from build123d import *

# Parameters (mm, degrees)
SKETCH_1_W          = 7
SKETCH_1_H          = 5
EXTRUDE_1_DEPTH     = 13
SKETCH_2_W          = 7
SKETCH_2_H          = 5
EXTRUDE_2_DEPTH     = 18.5
SKETCH_4_W          = 20
SKETCH_4_H          = 10
EXTRUDE_3_DEPTH     = 3
SKETCH_5_R          = 1.5
CUT_EXTRUDE_1_DEPTH = 34.559648389
FILLET_1_R          = 10
SKETCH_6_W          = 7
SKETCH_6_H          = 8
CUT_EXTRUDE_2_DEPTH = 0.1
CHAMFER_3_SIZE      = 2
CHAMFER_3_SIZE2     = 3


with BuildPart() as part:
    # 草图1 → 凸台-拉伸1 (new body)
    with BuildSketch(Plane(origin=(0, 0, 0), x_dir=(1, 0, 0), z_dir=(0, 1, 0))):
        Rectangle(SKETCH_1_W, SKETCH_1_H)
    extrude(amount=EXTRUDE_1_DEPTH)

    # 草图2 → 凸台-拉伸2 (add)
    with BuildSketch(Plane(origin=(0, 0, -2.5), x_dir=(-1, 0, 0), z_dir=(0, 0, -1))):
        with Locations((0, 10.5)):
            Rectangle(SKETCH_2_W, SKETCH_2_H)
    extrude(amount=EXTRUDE_2_DEPTH)

    # 草图4 → 凸台-拉伸3 (add)
    with BuildSketch(Plane(origin=(0, 0, -21), x_dir=(-1, 0, 0), z_dir=(0, 0, -1))):
        with Locations((0, 13)):
            Rectangle(SKETCH_4_W, SKETCH_4_H)
    extrude(amount=EXTRUDE_3_DEPTH)

    # 草图5 → 切除-拉伸1 (cut, through all)
    with BuildSketch(Plane(origin=(0, 0, -24), x_dir=(-1, 0, 0), z_dir=(0, 0, -1))):
        with Locations((-7, 13)):
            Circle(SKETCH_5_R)
        with Locations((7, 13)):
            Circle(SKETCH_5_R)
    extrude(amount=-CUT_EXTRUDE_1_DEPTH, mode=Mode.SUBTRACT)

    # 圆角1
    # the kernel refuses this fillet: 10 mm, written as the material it adds along each edge
    with BuildSketch(Plane(origin=(3.5, 13, -21), x_dir=(0, 1, 0), z_dir=(-1, 0, 0))) as fillet_1_piece_1:
        with BuildLine():
            CenterArc((10, -8.660254038), FILLET_1_R, 120, 60)
            Line((0, -8.660254038), (-0.2, -8.660254038))
            Line((-0.2, -8.660254038), (-0.2, 0))
            Line((-0.2, 0), (0, 0.2))
            ThreePointArc((0, 0.2), (2.5, 0.2), (4.9, 0.173205081))
            Line((4.9, 0.173205081), (5, 0))
        make_face()
    extrude(amount=7)

    # 草图6 → 切除-拉伸2 (cut)
    with BuildSketch(Plane(origin=(0, 0, -2.5), x_dir=(-1, 0, 0), z_dir=(0, 0, -1))):
        with Locations((0, 4)):
            Rectangle(SKETCH_6_W, SKETCH_6_H)
    extrude(amount=-CUT_EXTRUDE_2_DEPTH, mode=Mode.SUBTRACT)

    # 倒角3
    chamfer_3_edges = [part.edges().sort_by_distance(p)[0] for p in [
        (3.5, 0, 0.05),
        (-3.5, 0, 0.05),
    ]]
    chamfer_3_side = [part.faces().sort_by_distance(p)[0] for p in [
        (0, 0, 0.05),
    ]]
    chamfer(chamfer_3_edges, length=CHAMFER_3_SIZE, length2=CHAMFER_3_SIZE2, reference=chamfer_3_side[0])


solid = part.part
CAD build for the part. Positions are in the model's coordinates, mm. A direction names the side the tool comes from. Round coordinates to 2 decimals unless told otherwise and drop trailing zeros. Loops run counter-clockwise (first coordinate to the right, second up) from the corner with the lowest first, then second, coordinate; pieces in that order, holes last. Notation, with made-up numbers: (-34.5, 47.5) - (-2.5, 47.5) arc R21 ccw to (-2.5, 85.5) - close; hole circle Ø5 at (48, 38.25). An arc over 180 degrees is marked (long way). Put each result on its own line as item: value.
1. Two-plate mould, pull along X, no slides. Class faces 1 (the flat face through (2.5, 1.5, 0.1)), 2 (the flat face through (0, 4, -2.4)), 3 (the cylindrical face through (8.5, 13.07, -22.52)): released by +X, released by -X, zero draft, split by the parting line, or undercut.
Geometry check:
face 1: released by +X
face 2: zero draft
face 3: undercut
2. Slice it at C-C on y = 10. List the corners of the cut face in (x, z), and give its area (4 significant figures).
Geometry check:
outline: (-10, -24) - (10, -24) - (10, -21) - (3.5, -21) - (3.5, 2.5) - (-3.5, 2.5) - (-3.5, -21) - (-10, -21) - close
area: 224.5 mm²
3. Slice it at D-D on x = -2. List the corners of the cut face in (y, z), and give its area (3 significant figures).
Geometry check:
outline: (0.75, -2.4) - (8, -2.4) - (8, -24) - (18, -24) - (18, -21) arc R10 cw to (13, -12.34) - (13, 2.5) - (0.75, 2.5) - close
area: 196 mm²
4. 3-axis set-ups, long thin cutter, end or side, ignore diameter. For faces 4 (the flat face through (-3.5, 11, -9)), 5 (the flat face through (3.5, 11, -9)), 6 (the flat face through (0, 8, -15)), 7 (the flat face through (0, 13, -5)), 8 (the cylindrical face through (-5.5, 13.07, -22.52)): which of +Z, -Z, +X, -X, +Y, -Y reach the whole face in a straight line?
Geometry check:
face 4: +Z, -X, +Y, -Y
face 5: +Z, +X, +Y, -Y
face 6: -Z, +X, -X, -Y
face 7: +Z, +X, -X, +Y
face 8: +Z, -Z
5. Slice it at B-B on z = -22.25. List the corners of the cut face in (x, y).
Geometry check:
outline: (-10, 8) - (10, 8) - (10, 18) - (-10, 18) - close; hole circle Ø3 at (-7, 13); hole circle Ø3 at (7, 13)
6. Pin check, flat tips, straight feed: P1, Ø6, axis at y = 5, z = -4.5, coming from the -X side; P2, Ø6, axis at x = -3, z = -11, coming from the -Y side; P3, Ø3.5, axis at x = 1, y = 4.5, coming from the -Z side. Stop position of each tip, or through.
Geometry check:
P1: x = -3.5
P2: y = 8
P3: z = -2.4
7. Wall check: line 1 (Y direction, x = 7, z = -22.1); line 2 (X direction, y = 12.25, z = -3.25); line 3 (Z direction, x = 6, y = 10.75). Give the ranges that are in metal, low to high.
Geometry check:
line 1: 8 to 11.5, 14.5 to 18
line 2: -3.5 to 3.5
line 3: -24 to -21
8. Slice it at A-A on x = 7. List the corners of the cut face in (y, z), and give its area (3 significant figures).
Geometry check:
outline: (8, -24) - (11.5, -24) - (11.5, -21) - (8, -21) - close; (14.5, -24) - (18, -24) - (18, -21) - (14.5, -21) - close
area: 21.0 mm²
